Input: part model. Units: mm. Frame: model coordinates. A direction names the side the tool comes from. Give positions to 0.01 mm unless a question says otherwise; leave off trailing zeros. Loops run counter-clockwise (first coordinate to the right, second up) from the corner with the lowest first, then second, coordinate; pieces in that order, holes last. Notation, with made-up numbers: (7, 64.5) -> (53, 64.5) arc R18 ccw to (53, 87.5) -> close; hole circle Ø8 at (6, 47.5). An arc over 180 degrees is marked (long way). One line per question, with ' | ' between items.
from build123d import *

# Parameters (mm, degrees)
F0_R     = 3.81
F0_R_2   = 5.9944
F1_DEPTH = 5.08
F2_DEPTH = 76.2
F3_DEPTH = 76.2


with BuildPart() as f1:
    # F0 (on Front) → F1 (new body)
    with BuildSketch(Plane.XZ):
        with BuildLine():
            Line((36.615222, 3.8862), (4.730572, 3.8862))
            ThreePointArc((4.730572, 3.8862), (6.989429, 2.583681), (7.881685, 0.133605))
            ThreePointArc((7.881685, 0.133605), (1.736186, -2.876635), (3.124967, 3.82411))
            ThreePointArc((3.124967, 3.82411), (0.883733, 2.51609), (0, 0.0762))
            Line((0, 0.0762), (0, 0))
            Line((0, 0), (0, -18.171335))
            ThreePointArc((0, -18.171335), (20.650768, -31.684862), (41.3512, -18.247535))
            Line((41.3512, -18.247535), (41.3512, 0))
            Line((41.3512, 0), (41.3512, 0.0762))
            ThreePointArc((41.3512, 0.0762), (40.470217, 2.512788), (38.234685, 3.822555))
            ThreePointArc((38.234685, 3.822555), (40.291913, 2.466165), (41.08876, 0.134425))
            ThreePointArc((41.08876, 0.134425), (34.830493, -2.784837), (36.615222, 3.8862))
        make_face()
        with Locations((20.671425, -26.422268)):
            Circle(F0_R, mode=Mode.SUBTRACT)
        with Locations((20.671425, -15.165246)):
            Circle(F0_R_2, mode=Mode.SUBTRACT)
    extrude(amount=F1_DEPTH)

    # F0 (on Front) → F2 (join)
    with BuildSketch(Plane.XZ):
        with BuildLine():
            Line((4.730572, 3.8862), (3.81, 3.8862))
            ThreePointArc((3.81, 3.8862), (3.46608, 3.870646), (3.124967, 3.82411))
            ThreePointArc((3.124967, 3.82411), (1.736186, -2.876635), (7.881685, 0.133605))
            ThreePointArc((7.881685, 0.133605), (6.989429, 2.583681), (4.730572, 3.8862))
        make_face()
        with BuildLine():
            Line((37.5412, 3.8862), (36.615222, 3.8862))
            ThreePointArc((36.615222, 3.8862), (34.830493, -2.784837), (41.08876, 0.134425))
            ThreePointArc((41.08876, 0.134425), (40.291913, 2.466165), (38.234685, 3.822555))
            ThreePointArc((38.234685, 3.822555), (37.8894, 3.870255), (37.5412, 3.8862))
        make_face()
    extrude(amount=F2_DEPTH)

    # F0 (on Front) → F3 (join)
    with BuildSketch(Plane.XZ):
        with Locations((20.671425, -26.422268)):
            Circle(F0_R)
    extrude(amount=F3_DEPTH)


solid = f1.part
1. Section query D-D (z = -24.5). Output: boundary loops of the cut face in (x, y).
Determined:
outline: (4.17, -5.08) -> (17.38, -5.08) -> (17.38, -76.2) -> (23.96, -76.2) -> (23.96, -5.08) -> (37.22, -5.08) -> (37.22, 0) -> (4.17, 0) -> close
2. Section query C-C (y = -50). Output: boundary loops of the cut face in (x, z).
Determined:
outline: (3.12, 3.82) arc R3.81 ccw (long way) to (4.73, 3.89) -> (3.81, 3.89) arc R3.81 ccw to start; circle Ø7.62 at (20.67, -26.42); (36.62, 3.89) arc R3.81 ccw (long way) to (41.09, 0.13) arc R3.81 ccw to (38.23, 3.82) arc R3.81 ccw to (37.54, 3.89) -> close
3. Reachability of faces 1 (the cylindrical face through (24.305, -40.142, -25.278)), 2 (the flat face through (37, -76.2, 0)) from +Z, -Z, +X, -X, +Y, -Y: full face, straight path, thin tool, end or side. Return the list, or none.
Determined:
face 1: -Y | face 2: +Z, -Z, +X, -X, -Y
4. Section query B-B (z = -12.5). Output: boundary loops of the cut face in (x, y).
Determined:
outline: (0, -5.08) -> (15.3, -5.08) -> (15.3, 0) -> (0, 0) -> close; (26.04, -5.08) -> (41.35, -5.08) -> (41.35, 0) -> (26.04, 0) -> close
5. Ray query, line 1 along Y through (x, z) = (6, -25); line 2 along X through (y, z) = (-13, 2); line 3 along X through (y, z) = (-64, 0). Return the intervals inside material, ascending. Write a range as from..to.
Determined:
line 1: y = -5.08..0 | line 2: x = 0.75..7.39, 33.96..40.6 | line 3: x = 0.26..7.88, 33.47..41.09
6. Pull-direction query (X, two-part tool) for faces 3 (the cylindrical face through (20.29, -2.5, -31.68)), 4 (the cylindrical face through (16.253, -2.504, -11.114)), 5 (the flat face through (25, 0, -10)); classes: pulls with the +X half, pulls with the -X half, needs draft (parallel to the pull), parting line crosses it, or undercut.
Determined:
face 3: parting line crosses it | face 4: undercut | face 5: needs draft
7. Section query A-A (x = 23.5). Output: boundary loops of the cut face in (y, z).
Determined:
outline: (-76.2, -28.97) -> (-5.08, -28.97) -> (-5.08, -31.51) -> (0, -31.51) -> (0, -20.45) -> (-5.08, -20.45) -> (-5.08, -23.87) -> (-76.2, -23.87) -> close; (-5.08, -9.88) -> (0, -9.88) -> (0, 3.89) -> (-5.08, 3.89) -> close
8. Pin query (flat end, axial travel): P1, Ø1, axis at x = 6, y = -59, coming from the +Z side; P2, Ø2, axis at x = 7, z = -8, coming from the +Y side; P3, Ø1.5, axis at x = 19, y = -16.5, coming from the -Z side; P4, Ø2, axis at x = 14.5, y = -51.5, coming from the -Z side. Return the tip coordinate at first contact, or that it passes through.
Determined:
P1: stops at z = 3.67 | P2: stops at y = 0 | P3: stops at z = -30.12 | P4: passes through
